Input: dimensioned drawing with shaded views. Units: mm. Origin: part minimum x, y, z. A direction names the side the tool comes from. Round coordinates to 2 decimals unless told otherwise and drop trailing zeros. Write each loop counter-clockwise with the first axis right and the second up, starting at its lowest first coordinate (ties: lowest second). Pieces come first, ordered by that corner, then holes. Notation, with made-up numbers: (79.5, 23.5) -> (90.5, 23.5) arc R26 ccw to (90.5, 46.5) -> close; hole circle Ø1 at (78.5, 88). An arc over 180 degrees is marked (long way). Use one line per item in the form item = value. Start each with the question number.
1. Cut plane C-C, the plane y = 26. Return the cut outline in (x, z) (3 decimals).
2. Reachability of the marked faces 1, 2 and 3 from +Z, -Z, +X, -X, +Y, -Y: full face, straight path, thin tool, end or side. Return the list, or none.
3. Cut plane A-A, the plane z = 17.5. Return the cut outline in (x, y).
4. Line query: L1, parallel to Y at x = 33.5, z = 19; L2, parallel to Z at x = 3, y = 8 (3 decimals). Output: solid intervals per line, ascending.
5. Cut plane D-D, the plane z = 22.5. Return the cut outline in (x, y).
6. Cut plane B-B, the plane x = 8. Return the cut outline in (y, z) (3 decimals).
7. Pin query (flat end, axial travel): pin 1 Ø12.5 at (x, z) = (5.5, 25.5) entering from -Y; pin 2 Ø17.5 at (y, z) = (7, 27.5) entering from -X; pin 3 Ø12.5 at (y, z) = (11.5, 27) entering from +X. Return the tip coordinate at first contact, or that it passes through.
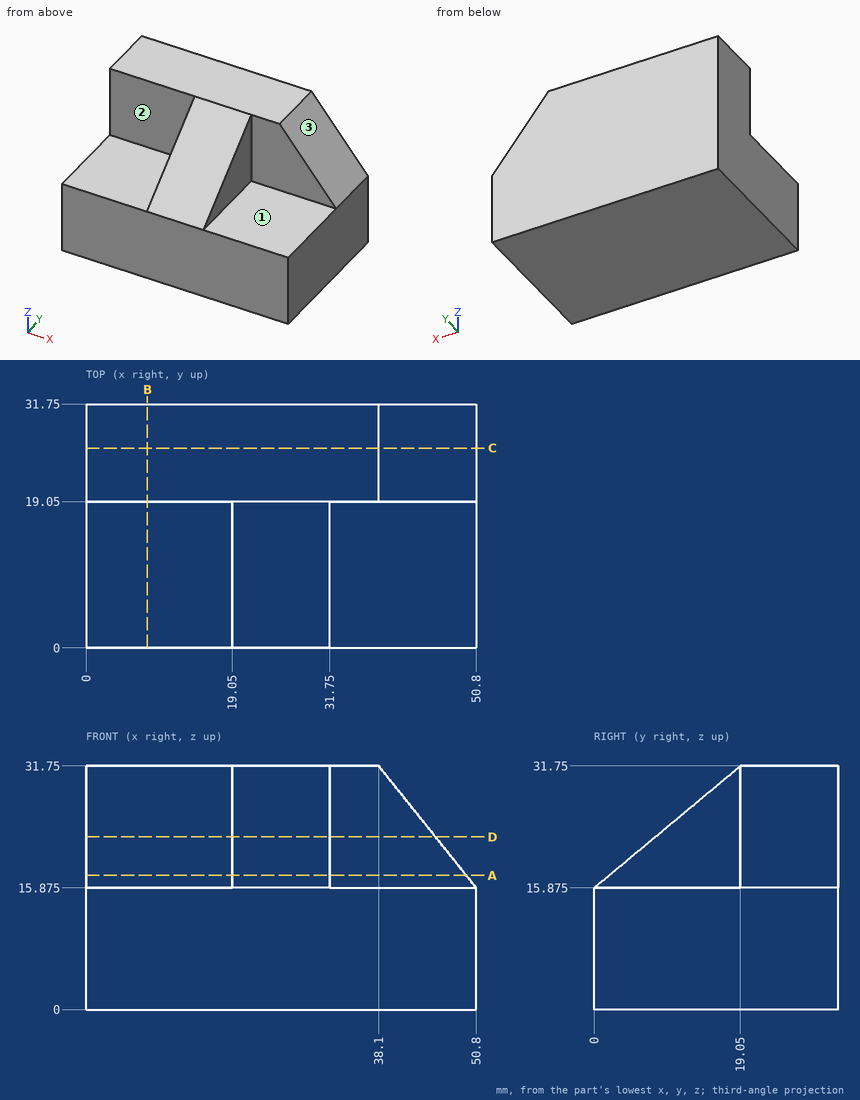
Outcome:
q1.outline = (0, 0) -> (50.8, 0) -> (50.8, 15.875) -> (38.1, 31.75) -> (0, 31.75) -> close
q2.face_1 = +Z, +X, -Y
q2.face_2 = +Z, -X, -Y
q2.face_3 = +Z, +X, +Y, -Y
q3.outline = (0, 19.05) -> (19.05, 19.05) -> (19.05, 1.95) -> (31.75, 1.95) -> (31.75, 19.05) -> (49.5, 19.05) -> (49.5, 31.75) -> (0, 31.75) -> close
q4.L1 = 19.05 to 31.75
q4.L2 = 0 to 15.875
q5.outline = (0, 19.05) -> (19.05, 19.05) -> (19.05, 7.95) -> (31.75, 7.95) -> (31.75, 19.05) -> (45.5, 19.05) -> (45.5, 31.75) -> (0, 31.75) -> close
q6.outline = (0, 0) -> (31.75, 0) -> (31.75, 31.75) -> (19.05, 31.75) -> (19.05, 15.875) -> (0, 15.875) -> close
q7.pin_1 = 19.05
q7.pin_2 = 19.05
q7.pin_3 = 31.75
